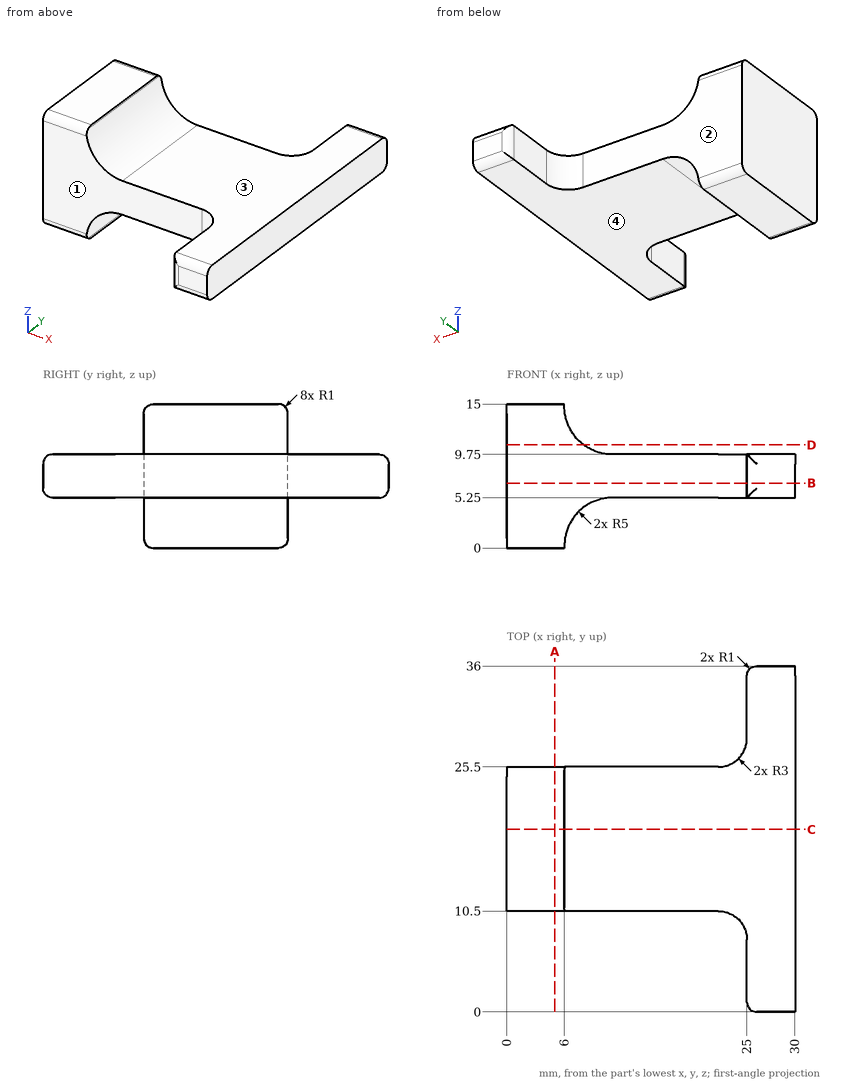
Geometry check sheet. Reference: drawing and pictorial views, mm from the part's lowest x, y, z. A direction names the side the tool comes from. Round coordinates to 2 decimals unless told otherwise and drop trailing zeros. Order: outer loops, then holes, each group sorted by start corner. A loop starts at its lowest first (then second) coordinate and runs counter-clockwise, first axis right, second up. Notation, with made-up numbers: (-25, 44.25) - (16, 44.25) arc R27 cw to (16, 76.25) - close; hole circle Ø7 at (-23.5, -19). An arc over 180 degrees is marked (long way). Use a Markdown table: item, result. Add a question column.
1) Section check C-C (y = 19). Record the cut outline in (x, z), then the cut area to 3 significant figures.
2) Thickness scan on line 1 along X through (y, z) = (5, 9.25); line 2 along Z through (x, y) = (20.5, 14); line 3 along Y through (x, z) = (13, 6.75). Record the ranges inside material, lowest first.
3) Section check A-A (x = 5). Record the cut outline in (y, z), then the cut area to 3 significant figures.
4) Section check B-B (z = 6.75). Record the cut outline in (x, y), then the cut area to 3 significant figures.
5) Section check D-D (z = 10.75). Record the cut outline in (x, y), then the cut area to 3 significant figures.
6) Gauge pin test, flat ends, axial feed: P1, Ø1.4, axis at y = 30.5, z = 7.5, coming from the -X side; P2, Ø5.5, axis at x = 20, y = 15, coming from the +Z side; P3, Ø9.5, axis at x = 17, y = 14.5, coming from the -Z side. Record the tip position at first contact, or that the pin passes through.
7) Set-up check for the marked faces 1, 2, 3 and 4: record each of +Z, -Z, +X, -X, +Y, -Y from which the full face is reachable in a straight line by a thin tool's end or side.
Established:
| question | item | result |
|---|---|---|
| 1 | outline | (0, 0) - (6, 0) - (6, 0.25) arc R5 cw to (11, 5.25) - (30, 5.25) - (30, 9.75) - (11, 9.75) arc R5 cw to (6, 14.75) - (6, 15) - (0, 15) - close |
| 1 | area | 209 mm2 |
| 2 | line 1 | 25 to 30 |
| 2 | line 2 | 5.25 to 9.75 |
| 2 | line 3 | 10.5 to 25.5 |
| 3 | outline | (10.5, 1) arc R1 ccw to (11.5, 0) - (24.5, 0) arc R1 ccw to (25.5, 1) - (25.5, 14) arc R1 ccw to (24.5, 15) - (11.5, 15) arc R1 ccw to (10.5, 14) - close |
| 3 | area | 224 mm2 |
| 4 | outline | (0, 10.5) - (22, 10.5) arc R3 cw to (25, 7.5) - (25, 1) arc R1 ccw to (26, 0) - (30, 0) - (30, 36) - (26, 36) arc R1 ccw to (25, 35) - (25, 28.5) arc R3 cw to (22, 25.5) - (0, 25.5) - close |
| 4 | area | 558 mm2 |
| 5 | outline | (0, 10.5) - (8, 10.5) - (8, 25.5) - (0, 25.5) - close |
| 5 | area | 120 mm2 |
| 6 | P1 | x = 25 |
| 6 | P2 | z = 9.75 |
| 6 | P3 | z = 5.25 |
| 7 | face 1 | +Z, -Z, -X, -Y |
| 7 | face 2 | +Z, -Z, -X, +Y |
| 7 | face 3 | +Z, +X, +Y, -Y |
| 7 | face 4 | -Z, +X, +Y, -Y |
